```python
from build123d import *

# Parameters (mm, degrees)
F0_W     = 151
F0_H     = 130
F1_DEPTH = 4.8
F2_W     = 99
F2_H     = 30
F2_R     = 1.55
F3_DEPTH = 4.8
F4_SIZE  = 20
F5_SIZE  = 20


with BuildPart() as f1:
    # F0 (on Front) → F1 (new body)
    with BuildSketch(Plane.XZ):
        Rectangle(F0_W, F0_H)
    extrude(amount=F1_DEPTH)

    # F2 (on face) → F3 (cut)
    with BuildSketch(Plane.XZ.offset(4.8)):
        Rectangle(F2_W, F2_H)
        with Locations((-59.5, 0)):
            Circle(F2_R)
        with Locations((59.5, 0)):
            Circle(F2_R)
        with Locations((-63.5, -55)):
            Circle(F2_R)
        with Locations((63.5, -55)):
            Circle(F2_R)
        with Locations((-58.5, -55)):
            Circle(F2_R)
        with Locations((58.5, -55)):
            Circle(F2_R)
        with Locations((-63.5, -26)):
            Circle(F2_R)
        with Locations((-58.5, -26)):
            Circle(F2_R)
        with Locations((63.5, -26)):
            Circle(F2_R)
        with Locations((58.5, -26)):
            Circle(F2_R)
        with Locations((65.5, 45)):
            Circle(F2_R)
        with Locations((-65.5, 45)):
            Circle(F2_R)
        with Locations((67.5, -16)):
            Circle(F2_R)
        with Locations((-67.5, -16)):
            Circle(F2_R)
        with Locations((10.5, 45)):
            Circle(F2_R)
        with Locations((-10.5, 45)):
            Circle(F2_R)
        with Locations((0.5, 26)):
            Circle(F2_R)
    extrude(amount=-F3_DEPTH, mode=Mode.SUBTRACT)

    # F4
    f4_edges = [f1.edges().sort_by_distance(p)[0] for p in [
        (-75.5, -2.4, 65),
    ]]
    chamfer(f4_edges, length=F4_SIZE)

    # F5
    f5_edges = [f1.edges().sort_by_distance(p)[0] for p in [
        (75.5, -2.4, 65),
    ]]
    chamfer(f5_edges, length=F5_SIZE)


solid = f1.part
```
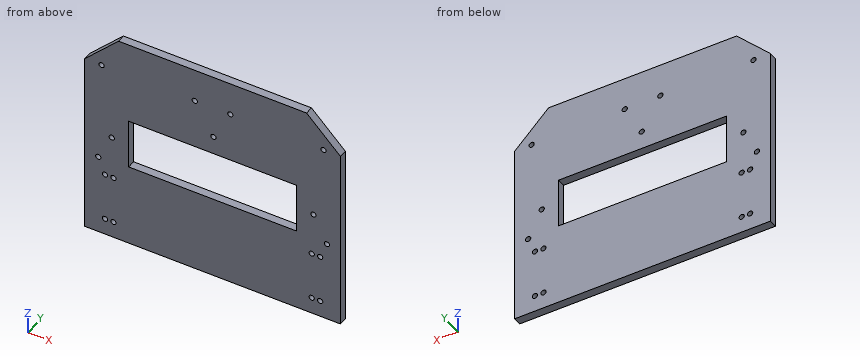
Verification items for the finished model (mm, model axes). Coordinates: 2 decimals unless noted, no trailing zeros. Order: outer loops, then holes, each group sorted by start corner. A loop starts at its lowest first (then second) coordinate and runs counter-clockwise, first axis right, second up. Notation, with made-up numbers: (60.25, 66) -> (76.25, 66) arc R13 cw to (76.25, 81) -> close; hole circle Ø1 at (28, 66). An arc over 180 degrees is marked (long way). Put each result on its own line as item: value. Start each with the question number.
1) Cross-section at A-A (z = 5.5). Enter the section's corners in (x, y), plus the area to 3 significant figures.
2) Cross-section at B-B (y = -0.8). State how many separate pieces and enclosed holes the cut face has, plus the area to 3 significant figures.
3) Go/stop test with a flat-tipped pin: pin 1 (5 mm diameter, centred on x = 67.5, z = -16, fed in from +Y). Record where the tip stops, or that it passes through.
4) Material ranges on L1, parallel to Z at x = 10.5, y = -1.4; L2, parallel to Z at x = -16.5, y = -3.95; L3, parallel to X at y = -3.45, z = -17, recorded low to high.
5) Cross-section at C-C (x = -23). Enter the section's corners in (y, z).
6) Cross-section at D-D (z = 55). Enter the section's corners in (x, y), plus the area to 3 significant figures.
Geometry check:
1. outline: (-75.5, -4.8) -> (-49.5, -4.8) -> (-49.5, 0) -> (-75.5, 0) -> close; (49.5, -4.8) -> (75.5, -4.8) -> (75.5, 0) -> (49.5, 0) -> close
1. area: 250 mm^2
2. separate pieces: 1
2. enclosed holes: 18
2. area: 16,100 mm^2
3. pin 1: stops at y = 0
4. L1: z = -65 to -15, 15 to 43.45, 46.55 to 65
4. L2: z = -65 to -15, 15 to 65
4. L3: x = -75.5 to -68.68, -66.32 to 66.32, 68.68 to 75.5
5. outline: (-4.8, -65) -> (0, -65) -> (0, -15) -> (-4.8, -15) -> close; (-4.8, 15) -> (0, 15) -> (0, 65) -> (-4.8, 65) -> close
6. outline: (-65.5, -4.8) -> (65.5, -4.8) -> (65.5, 0) -> (-65.5, 0) -> close
6. area: 629 mm^2
